Can you work these out from the drawing? Everything is in mm from the part's minimum corner. Coordinates: 2 decimals unless noted, no trailing zeros. Write each loop counter-clockwise with the first axis right and the second up, starting at its lowest first coordinate (ties: lowest second). Pieces come first, ordered by that corner, then holes. Notation, with made-up numbers: (-10, -35.5) - (24, -35.5) arc R22 ccw to (24, -28.5) - close; hole circle Ø2 at (-16.5, 72). An arc over 180 degrees is marked (long way). One line per question, with ' | ' between items. Start each with the question number.
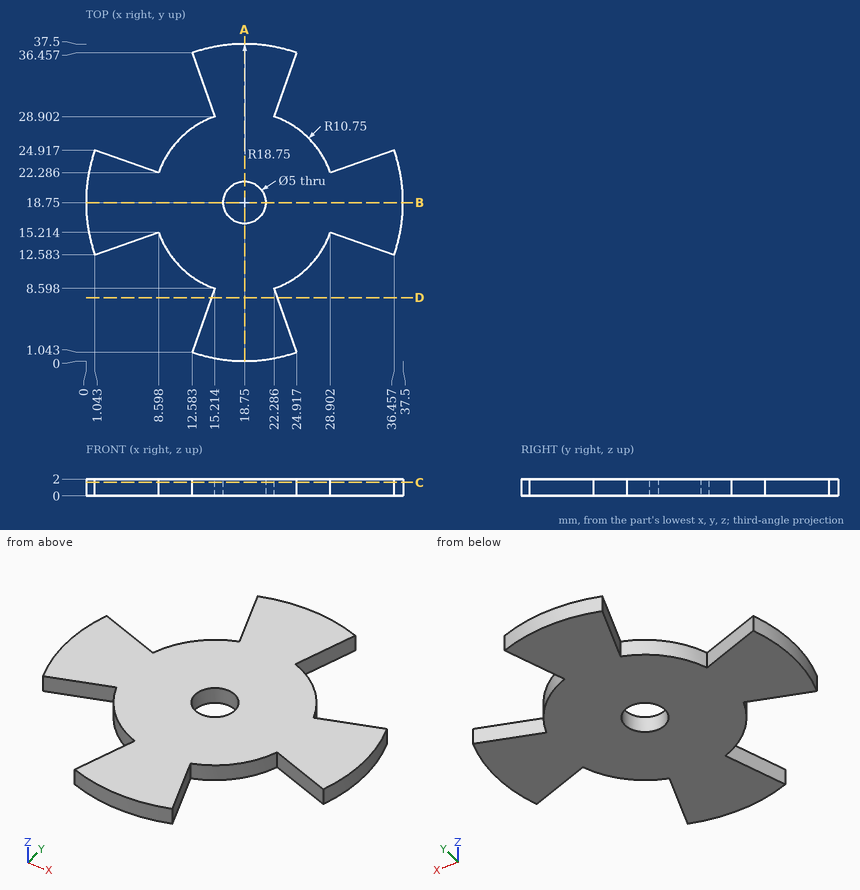
(1) If we section it at A-A on x = 18.75: List the corners of the cut face in (y, z) for me.
(2) I'm going to push flat-ended pins straight in: pin 1 (1 mm diameter, centred on y = 14, z = 1, fed in from +X); pin 2 (6 mm diameter, centred on x = 32, y = 8, fed in from -Z). Where does each tip first touch, or does it pass through?
(3) If we section it at D-D on y = 7.5: List the corners of the cut face in (x, z) for me, plus the area to 3 significant figures.
(4) If we section it at C-C on z = 1.6: List the corners of the cut face in (x, y) for me.
(5) If I drill on probe 1 along Y at (x, z) = (18.75, 1.6); probe 2 along Y at (x, z) = (16, 0.65); probe 3 along X at (y, z) = (27.5, 1.2) (1 decimal), over which ranges is the centre line in solid material (lowest first)?
Values:
1) outline: (0, 0) - (16.25, 0) - (16.25, 2) - (0, 2) - close; (21.25, 0) - (37.5, 0) - (37.5, 2) - (21.25, 2) - close
2) pin 1: x = 37.01 | pin 2: through
3) outline: (14.83, 0) - (22.67, 0) - (22.67, 2) - (14.83, 2) - close | area: 15.7 mm2
4) outline: (1.04, 12.58) - (8.6, 15.21) arc R10.75 ccw to (15.21, 8.6) - (12.58, 1.04) arc R18.75 ccw to (24.92, 1.04) - (22.29, 8.6) arc R10.75 ccw to (28.9, 15.21) - (36.46, 12.58) arc R18.75 ccw to (36.46, 24.92) - (28.9, 22.29) arc R10.75 ccw to (22.29, 28.9) - (24.92, 36.46) arc R18.75 ccw to (12.58, 36.46) - (15.21, 28.9) arc R10.75 ccw to (8.6, 22.29) - (1.04, 24.92) arc R18.75 ccw to start; hole circle Ø5 at (18.75, 18.75)
5) probe 1: 0 to 16.25, 21.25 to 37.5 | probe 2: 0.2 to 37.3 | probe 3: 12.5 to 25
